```python
from build123d import *

# Parameters (mm, degrees)
SKETCH1_R           = 2.032
SKETCH1_W           = 33.02
SKETCH1_H           = 52.3843179
BOSS_EXTRUDE1_DEPTH = 3.175
SKETCH1_3_R         = 2.032
SKETCH1_3_R_2       = 1.524
BOSS_EXTRUDE2_DEPTH = 7.62
SKETCH1_4_R         = 1.524
BOSS_EXTRUDE3_DEPTH = 9.271
SKETCH2_W           = 6.35
SKETCH2_H           = 52.3843179
CUT_EXTRUDE1_DEPTH  = 9.271


with BuildPart() as part:
    # Sketch1 → Boss-Extrude1 (new body)
    with BuildSketch(Plane.XY):
        Polygon((53.34, 68.199), (53.34, 65.786), (53.34, 0), (0, 0), (0, 65.786), (12.7, 65.786), (12.7, 68.199), (45.72, 68.199), align=None)
        with Locations((45.72, 65.786)):
            Circle(SKETCH1_R, mode=Mode.SUBTRACT)
        with Locations((17.653, 65.786)):
            Circle(SKETCH1_R, mode=Mode.SUBTRACT)
        with Locations((2.413, 13.589)):
            Circle(SKETCH1_R, mode=Mode.SUBTRACT)
        with Locations((50.927, 13.589)):
            Circle(SKETCH1_R, mode=Mode.SUBTRACT)
        with Locations((29.21, 31.18869335)):
            Rectangle(SKETCH1_W, SKETCH1_H, mode=Mode.SUBTRACT)
    extrude(amount=BOSS_EXTRUDE1_DEPTH)

    # Sketch1<3> → Boss-Extrude2 (add)
    # profile 1 of 4: a face of its own
    with BuildSketch(Plane.XY):
        with Locations(Location((17.653, 65.786, 0), (0, 0, 180))):
            Circle(SKETCH1_3_R)
        with Locations(Location((17.653, 65.786, 0), (0, 0, 180))):
            Circle(SKETCH1_3_R_2, mode=Mode.SUBTRACT)
    # profile 2 of 4: a face of its own
    with BuildSketch(Plane.XY):
        with Locations(Location((45.72, 65.786, 0), (0, 0, 180))):
            Circle(SKETCH1_3_R)
        with Locations(Location((45.72, 65.786, 0), (0, 0, 180))):
            Circle(SKETCH1_3_R_2, mode=Mode.SUBTRACT)
    # profile 3 of 4: a face of its own
    with BuildSketch(Plane.XY):
        with Locations(Location((50.927, 13.589, 0), (0, 0, 180))):
            Circle(SKETCH1_3_R)
        with Locations(Location((50.927, 13.589, 0), (0, 0, 180))):
            Circle(SKETCH1_3_R_2, mode=Mode.SUBTRACT)
    # profile 4 of 4: a face of its own
    with BuildSketch(Plane.XY):
        with Locations(Location((2.413, 13.589, 0), (0, 0, 180))):
            Circle(SKETCH1_3_R)
        with Locations(Location((2.413, 13.589, 0), (0, 0, 180))):
            Circle(SKETCH1_3_R_2, mode=Mode.SUBTRACT)
    extrude(amount=BOSS_EXTRUDE2_DEPTH)

    # Sketch1<4> → Boss-Extrude3 (add)
    with BuildSketch(Plane.XY):
        with Locations((2.413, 13.589)):
            Circle(SKETCH1_4_R)
        with Locations((17.653, 65.786)):
            Circle(SKETCH1_4_R)
        with Locations((45.72, 65.786)):
            Circle(SKETCH1_4_R)
        with Locations((50.927, 13.589)):
            Circle(SKETCH1_4_R)
    extrude(amount=BOSS_EXTRUDE3_DEPTH)

    # Sketch2 → Cut-Extrude1 (cut)
    with BuildSketch(Plane.XY.offset(3.175)):
        with Locations((9.525, 31.18869335)):
            Rectangle(SKETCH2_W, SKETCH2_H)
        Polygon((45.72, 57.3808523), (45.72, 61.1908523), (6.35, 61.1908523), (6.35, 57.3808523), (12.7, 57.3808523), align=None)
    extrude(amount=-CUT_EXTRUDE1_DEPTH, mode=Mode.SUBTRACT)


solid = part.part
```
Could you check a few things on this model? Use its own coordinates, in mm. A direction names the side the tool comes from. Round coordinates to 2 decimals unless told otherwise and drop trailing zeros. Order: outer loops, then holes, each group sorted by start corner. A loop starts at its lowest first (then second) coordinate and runs counter-clockwise, first axis right, second up. Notation, with made-up numbers: (2, 44.25) -> (29, 44.25) arc R31 ccw to (29, 72.25) -> close; hole circle Ø3 at (52, 43). An arc over 180 degrees is marked (long way). One line per question, with ' | ' between items.
Q1. Which directions (+Z, -Z, +X, -X, +Y, -Y) give clear straight access to the entire face, cutting with the end or side of a thin tool? Please do faces 1 (the face through (51, 14, 9.271)), 2 (the face through (50, 12, 7.62)).
Computed values:
face 1: +Z, +X, -X, +Y, -Y | face 2: +Z
Q2. If I drill on line 1 (X direction, y = 12, z = 2); line 2 (Y direction, x = 35.5, z = 0.75); line 3 (X direction, y = 65, z = 5.5), over which ranges is the centre line in solid material (lowest first)? Write a range as from..to.
Computed values:
line 1: 0..6.35, 45.72..53.34 | line 2: 0..5, 61.19..68.2 | line 3: 15.78..19.53, 43.85..47.59
Q3. I'm going to push flat-ended pins straight in: pin 1 (3 mm diameter, centred on y = 32.5, z = 3, fed in from -X); pin 2 (16 mm diameter, centred on x = 30, y = 21.5, fed in from +Z); pin 3 (2.5 mm diameter, centred on x = 8.5, z = 2.5, fed in from +Y); pin 4 (0.7 mm diameter, centred on y = 67.5, z = 1.5, fed in from -X). Where does each tip first touch, or does it pass through?
Computed values:
pin 1: x = 0 | pin 2: through | pin 3: y = 65.79 | pin 4: x = 12.7
Q4. We'd pull the mould along Y, two halves only. Please class faces 3 (the face through (18, 66, 9.271)), 4 (the face through (26, 61.191, 2)), 5 (the face through (47.174, 66.244, 8.434)), 6 (the face through (27, 0, 2)): released by +Y, released by -Y, zero draft, split by the parting line, or undercut.
Computed values:
face 3: zero draft | face 4: undercut | face 5: split by the parting line | face 6: released by -Y
Q5. If we section it at D-D on z = 5: Write out the boundary of the cut face in (x, y) (3 decimals), plus the area to 3 significant figures.
Computed values:
outline: circle Ø4.064 at (2.413, 13.589); circle Ø4.064 at (17.653, 65.786); circle Ø4.064 at (45.72, 65.786); circle Ø4.064 at (50.927, 13.589) | area: 51.9 mm²
Q6. If we section it at B-B on y = 28: Write out the boundary of the cut face in (x, z) (3 decimals).
Computed values:
outline: (0, 0) -> (6.35, 0) -> (6.35, 3.175) -> (0, 3.175) -> close; (45.72, 0) -> (53.34, 0) -> (53.34, 3.175) -> (45.72, 3.175) -> close
Q7. If we section it at A-A on x = 13.5: Write out the boundary of the cut face in (y, z) (3 decimals), plus the area to 3 significant figures.
Computed values:
outline: (0, 0) -> (4.997, 0) -> (4.997, 3.175) -> (0, 3.175) -> close; (61.191, 0) -> (68.199, 0) -> (68.199, 3.175) -> (61.191, 3.175) -> close | area: 38.1 mm²
Q8. If we section it at C-C on z = 1.5: Write out the boundary of the cut face in (x, y).
Computed values:
outline: (0, 0) -> (53.34, 0) -> (53.34, 68.2) -> (12.7, 68.2) -> (12.7, 65.79) -> (0, 65.79) -> close; hole (6.35, 5) -> (45.72, 5) -> (45.72, 61.19) -> (6.35, 61.19) -> close
